```python
from build123d import *

# Parameters (mm, degrees)
AUFSATZ_LINEAR_AUSTRAGEN1_DEPTH = 4
SKIZZE2_R                       = 3
SCHNITT_LINEAR_AUSTRAGEN1_DEPTH = 7
VERRUNDUNG1_R                   = 4
SKIZZE3_R                       = 1.55
SCHNITT_LINEAR_AUSTRAGEN2_DEPTH = 10.881295462
FASE1_SIZE                      = 0.5


with BuildPart() as part:
    # Skizze1 → Aufsatz-Linear austragen1 (new, symmetric)
    with BuildSketch(Plane.XY):
        Polygon((-8, 0), (8, 0), (8, 8), (0, 8), (0, 3.8), (-8, 3.8), align=None)
    extrude(amount=AUFSATZ_LINEAR_AUSTRAGEN1_DEPTH, both=True)

    # Skizze2 → Schnitt-Linear austragen1 (cut)
    with BuildSketch(Plane(origin=(8, 0, 0), x_dir=(0, 0, -1), z_dir=(1, 0, 0))):
        with Locations(Location((0, 4, 0), (0, 0, 90))):
            Circle(SKIZZE2_R)
    extrude(amount=-SCHNITT_LINEAR_AUSTRAGEN1_DEPTH, mode=Mode.SUBTRACT)

    # Verrundung1
    verrundung1_edges = [part.edges().sort_by_distance(p)[0] for p in [
        (-8, 1.9, -4),
        (-8, 1.9, 4),
    ]]
    fillet(verrundung1_edges, radius=VERRUNDUNG1_R - 0.0001)  # a hair under: the kernel refuses the full size

    # Skizze3 → Schnitt-Linear austragen2 (cut, through all)
    with BuildSketch(Plane(origin=(0, 3.8, 0), x_dir=(1, 0, 0), z_dir=(0, 1, 0))):
        with Locations(Location((-4, 0, 0), (0, 0, 180))):
            Circle(SKIZZE3_R)
    extrude(amount=-SCHNITT_LINEAR_AUSTRAGEN2_DEPTH, mode=Mode.SUBTRACT)

    # Fase1
    fase1_edges = [part.edges().sort_by_distance(p)[0] for p in [
        (-2.45, 3.8, 0),
    ]]
    chamfer(fase1_edges, length=FASE1_SIZE)


solid = part.part
```
CAD build for the part. Positions are in the model's coordinates, mm. A direction names the side the tool comes from. Coordinates: 2 decimals unless noted, no trailing zeros. Order: outer loops, then holes, each group sorted by start corner. A loop starts at its lowest first (then second) coordinate and runs counter-clockwise, first axis right, second up.
(1) Mould opens along Z. For faces 1 (the face through (4, 8, 0)), 2 (the face through (5, 1, 0)), 3 (the face through (-6.797, 1.873, 2.859)), 4 (the face through (1, 4, 0)) say: released by +Z, released by -Z, zero draft, split by the parting line, or undercut.
Solution:
face 1: zero draft
face 2: undercut
face 3: released by +Z
face 4: undercut
(2) Saw through at C-C, the plane y = 5.5. Write the cut outline in (x, z).
Solution:
outline: (0, -4) - (8, -4) - (8, -2.6) - (1, -2.6) - (1, 2.6) - (8, 2.6) - (8, 4) - (0, 4) - close
(3) Drill centre lines: L1, parallel to Z at x = -4, y = 2.4; L2, parallel to Z at x = 3.75, y = 4; L3, parallel to X at y = 7, z = -3.25. Where is each one in solid material? Low to high.
Solution:
L1: z = -4 to -1.55, 1.55 to 4
L2: z = -4 to -3, 3 to 4
L3: x = 0 to 8
(4) Saw through at B-B, the plane x = -0.25. Write the cut outline in (y, z), and give its area (3 significant figures).
Solution:
outline: (0, -4) - (3.8, -4) - (3.8, 4) - (0, 4) - close
area: 30.4 mm2
(5) Saw through at D-D, the plane z = 2.75. Write the cut outline in (x, y), and give its area (3 significant figures).
Solution:
outline: (-6.9, 0) - (8, 0) - (8, 2.8) - (1, 2.8) - (1, 5.2) - (8, 5.2) - (8, 8) - (0, 8) - (0, 3.8) - (-6.9, 3.8) - close
area: 73.5 mm2
(6) Which spindle directions (+Z, -Z, +X, -X, +Y, -Y) get a long thin tool onto all of the face, cutting with end or side? Do faces 5 (the face through (0, 6, 0)), 6 (the face through (-2.45, 1.67, 0.07)). Say none if no direction does.
Solution:
face 5: +Z, -Z, -X, +Y
face 6: +Y, -Y
(7) Pin check, flat tips, straight feed: pin 1 Ø3.5 at (y, z) = (4, 0) entering from +X; pin 2 Ø2 at (y, z) = (5, -0.5) entering from -X; pin 3 Ø2.5 at (x, z) = (-4.5, 1.5) entering from +Y; pin 4 Ø2 at (x, y) = (-5.5, 5.5) entering from -Z. Stop position of each tip, or through.
Solution:
pin 1: stops at x = 1
pin 2: stops at x = 0
pin 3: stops at y = 3.8
pin 4: passes through
